The model under review builds one solid part; all positions refer to its coordinate system, in mm. Round coordinates to 2 decimals unless told otherwise and drop trailing zeros. Write each loop counter-clockwise with the first axis right and the second up, starting at its lowest first coordinate (ties: lowest second). Pieces come first, ordered by that corner, then holes. Notation, with made-up numbers: (7.25, 72) -> (47.25, 72) arc R30 ccw to (47.25, 109) -> close; hole circle Ø1 at (-13, -3.5). An arc over 180 degrees is marked (long way). Return JSON: item names as keys, results as strings. Group by question number.
1. Clearance check with a flat-ended pin moving along its axis: P1, Ø3.5, axis at x = 52.5, z = 15, coming from the +Y side. State where the tip first meets the part, or that it passes through.
2. For line 1 along X through (y, z) = (1.95, 0); line 2 along Z through (x, y) = (21.5, 1.7); line 3 along X through (y, z) = (1.5, 14), list the stretches that pass through material, from the lowest coordinate up. Write a range as from..to.
3. Take a section at A-A, the plane z = 12.5. Write out the cut boundary in (x, y), then the cut area to 3 significant figures.
4. Take a section at D-D, the plane z = 0. Write out the cut boundary in (x, y).
5. Take a section at C-C, the plane y = 0.95. Write out the cut boundary in (x, z).
6. Take a section at B-B, the plane x = -22.5. Write out the cut boundary in (y, z).
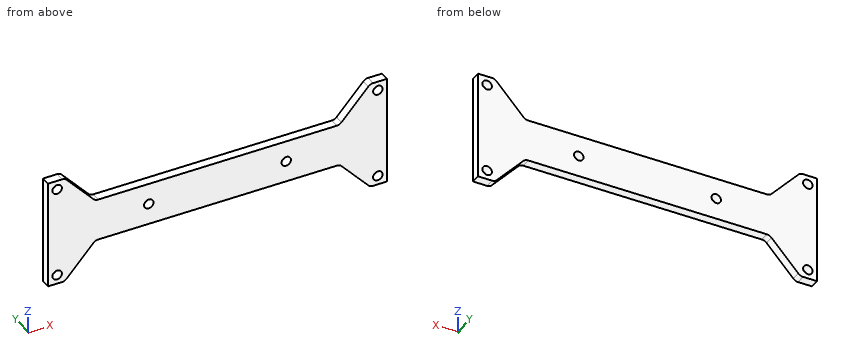
from build123d import *

# Parameters (mm, degrees)
SKETCH_1_W          = 111
SKETCH_1_H          = 36
SKETCH_1_R          = 1.55
EXTRUDE_1_DEPTH     = 3
CUT_EXTRUDE_1_DEPTH = 59.423026282
FILLET_2_R          = 2.1


with BuildPart() as part:
    # ｽｹｯﾁ1 → ﾎﾞｽ - 押し出し1 (new body)
    with BuildSketch(Plane(origin=(0, 0, 0), x_dir=(1, 0, 0), z_dir=(0, 1, 0))):
        Rectangle(SKETCH_1_W, SKETCH_1_H)
        with Locations(Location((-52.5, 15, 0), (0, 0, 270))):
            Circle(SKETCH_1_R, mode=Mode.SUBTRACT)
        with Locations(Location((-52.5, -15, 0), (0, 0, 270))):
            Circle(SKETCH_1_R, mode=Mode.SUBTRACT)
        with Locations(Location((52.5, -15, 0), (0, 0, 270))):
            Circle(SKETCH_1_R, mode=Mode.SUBTRACT)
        with Locations(Location((52.5, 15, 0), (0, 0, 270))):
            Circle(SKETCH_1_R, mode=Mode.SUBTRACT)
        with Locations(Location((-22.5, 0, 0), (0, 0, 270))):
            Circle(SKETCH_1_R, mode=Mode.SUBTRACT)
        with Locations(Location((22.5, 0, 0), (0, 0, 270))):
            Circle(SKETCH_1_R, mode=Mode.SUBTRACT)
    extrude(amount=EXTRUDE_1_DEPTH)

    # ｽｹｯﾁ2 → ｶｯﾄ - 押し出し1 (cut, through all)
    with BuildSketch(Plane(origin=(0, 3, 0), x_dir=(1, 0, 0), z_dir=(0, 1, 0))):
        Polygon((-50, 18), (-40, 7), (40, 7), (50, 18), align=None)
        Polygon((50, -18), (-50, -18), (-40, -7), (40, -7), align=None)
    extrude(amount=-CUT_EXTRUDE_1_DEPTH, mode=Mode.SUBTRACT)

    # ﾌｨﾚｯﾄ2
    fillet_2_edges = [part.edges().sort_by_distance(p)[0] for p in [
        (-50, 1.5, -18),
        (50, 1.5, -18),
        (40, 1.5, -7),
        (-40, 1.5, -7),
        (40, 1.5, 7),
        (50, 1.5, 18),
        (-50, 1.5, 18),
        (-40, 1.5, 7),
    ]]
    fillet(fillet_2_edges, radius=FILLET_2_R)


solid = part.part
Output:
{
 "1": {"P1": "stops at y = 3"},
 "2": {"line 1": "x = -55.5..-24.05, -20.95..20.95, 24.05..55.5", "line 2": "z = -7..-1.18, 1.18..7", "line 3": "x = -55.5..-53.68, -51.32..-46.36, 46.36..51.32, 53.68..55.5"},
 "3": {"outline": "(-55.5, 0) -> (-45, 0) -> (-45, 3) -> (-55.5, 3) -> close; (45, 0) -> (55.5, 0) -> (55.5, 3) -> (45, 3) -> close", "area": "63.0 mm^2"},
 "4": {"outline": "(-55.5, 0) -> (-24.05, 0) -> (-24.05, 3) -> (-55.5, 3) -> close; (-20.95, 0) -> (20.95, 0) -> (20.95, 3) -> (-20.95, 3) -> close; (24.05, 0) -> (55.5, 0) -> (55.5, 3) -> (24.05, 3) -> close"},
 "5": {"outline": "(-55.5, -18) -> (-50.93, -18) arc R2.1 ccw to (-49.38, -17.31) -> (-40.62, -7.69) arc R2.1 cw to (-39.07, -7) -> (39.07, -7) arc R2.1 cw to (40.62, -7.69) -> (49.38, -17.31) arc R2.1 ccw to (50.93, -18) -> (55.5, -18) -> (55.5, 18) -> (50.93, 18) arc R2.1 ccw to (49.38, 17.31) -> (40.62, 7.69) arc R2.1 cw to (39.07, 7) -> (-39.07, 7) arc R2.1 cw to (-40.62, 7.69) -> (-49.38, 17.31) arc R2.1 ccw to (-50.93, 18) -> (-55.5, 18) -> close; hole circle Ø3.1 at (-52.5, -15); hole circle Ø3.1 at (-52.5, 15); hole circle Ø3.1 at (-22.5, 0); hole circle Ø3.1 at (22.5, 0); hole circle Ø3.1 at (52.5, -15); hole circle Ø3.1 at (52.5, 15)"},
 "6": {"outline": "(0, -7) -> (3, -7) -> (3, -1.55) -> (0, -1.55) -> close; (0, 1.55) -> (3, 1.55) -> (3, 7) -> (0, 7) -> close"}
}
